from build123d import *

# Parameters (mm, degrees)
SKETCH1_R           = 251.5
BOSS_EXTRUDE1_DEPTH = 3
SKETCH2_R           = 2.5
CUT_EXTRUDE1_DEPTH  = 5
SKETCH4_R           = 2.5
CUT_EXTRUDE3_DEPTH  = 5
SKETCH5_W           = 73.96870399
SKETCH5_H           = 122
SKETCH5_W_2         = 122.237238898
SKETCH5_H_2         = 252
CUT_EXTRUDE4_DEPTH  = 10
FILLET1_R           = 2


with BuildPart() as part:
    # Sketch1 → Boss-Extrude1 (new body)
    with BuildSketch(Plane(origin=(0, 0, 0), x_dir=(1, 0, 0), z_dir=(0, 1, 0))):
        with Locations(Location((0, 0, 0), (0, 0, 270))):
            Circle(SKETCH1_R)
    extrude(amount=BOSS_EXTRUDE1_DEPTH)

    # Sketch2 → Cut-Extrude1 (cut)
    with BuildSketch(Plane(origin=(0, 3, 0), x_dir=(1, 0, 0), z_dir=(0, 1, 0))):
        with Locations(Location((-136, 118, 0), (0, 0, 270))):
            Circle(SKETCH2_R)
        with Locations(Location((136, 118, 0), (0, 0, 270))):
            Circle(SKETCH2_R)
        with Locations(Location((136, -118, 0), (0, 0, 270))):
            Circle(SKETCH2_R)
        with Locations(Location((-136, -118, 0), (0, 0, 270))):
            Circle(SKETCH2_R)
    extrude(amount=-CUT_EXTRUDE1_DEPTH, mode=Mode.SUBTRACT)

    # Sketch4 → Cut-Extrude3 (cut)
    with BuildSketch(Plane(origin=(0, 3, 0), x_dir=(1, 0, 0), z_dir=(0, 1, 0))):
        with Locations(Location((0, 242.5, 0), (0, 0, 270))):
            Circle(SKETCH4_R)
        with Locations(Location((142.537923681, 196.186621136, 0), (0, 0, 270))):
            Circle(SKETCH4_R)
        with Locations(Location((230.631205202, 74.936621136, 0), (0, 0, 270))):
            Circle(SKETCH4_R)
        with Locations(Location((230.631205202, -74.936621136, 0), (0, 0, 270))):
            Circle(SKETCH4_R)
        with Locations(Location((142.537923681, -196.186621136, 0), (0, 0, 270))):
            Circle(SKETCH4_R)
        with Locations(Location((0, -242.5, 0), (0, 0, 270))):
            Circle(SKETCH4_R)
        with Locations(Location((-142.537923681, -196.186621136, 0), (0, 0, 270))):
            Circle(SKETCH4_R)
        with Locations(Location((-230.631205202, -74.936621136, 0), (0, 0, 270))):
            Circle(SKETCH4_R)
        with Locations(Location((-230.631205202, 74.936621136, 0), (0, 0, 270))):
            Circle(SKETCH4_R)
        with Locations(Location((-142.537923681, 196.186621136, 0), (0, 0, 270))):
            Circle(SKETCH4_R)
    extrude(amount=-CUT_EXTRUDE3_DEPTH, mode=Mode.SUBTRACT)

    # Sketch5 → Cut-Extrude4 (cut)
    with BuildSketch(Plane(origin=(0, 3, 0), x_dir=(1, 0, 0), z_dir=(0, 1, 0))):
        with Locations((-225.484351995, 0)):
            Rectangle(SKETCH5_W, SKETCH5_H)
        with Locations((225.618619449, 0)):
            Rectangle(SKETCH5_W_2, SKETCH5_H_2)
    extrude(amount=-CUT_EXTRUDE4_DEPTH, mode=Mode.SUBTRACT)

    # Fillet1
    fillet1_edges = [part.edges().sort_by_distance(p)[0] for p in [
        (-188.5, 1.5, -61),
        (-243.990266199, 1.5, 61),
        (-188.5, 1.5, 61),
        (-243.990266199, 1.5, -61),
        (164.5, 1.5, 126),
        (217.660860055, 1.5, -126),
        (164.5, 1.5, -126),
        (217.660860055, 1.5, 126),
    ]]
    fillet(fillet1_edges, radius=FILLET1_R)


solid = part.part
Source: CAD feature listing. Evaluate the final solid. Frame: model axes, mm. Give positions to 0.01 mm unless a question says otherwise; leave off trailing zeros. Write each loop counter-clockwise with the first axis right and the second up, starting at its lowest first coordinate (ties: lowest second). Pieces come first, ordered by that corner, then holes. Notation, with made-up numbers: (8.5, 39) -> (66.5, 39) arc R33 ccw to (66.5, 75) -> close; hole circle Ø10 at (-17.5, 7.25). An arc over 180 degrees is marked (long way). Write item = value, one per line.
Q1. Cut plane A-A on y = 1.8. State how many separate pieces and enclosed holes the cut face has, then the cut area to 3 significant figures.
Here are the results:
separate_pieces = 1
enclosed_holes = 12
area = 172,000 mm²
Q2. Mould query, pull axis Y, two halves, no side actions, for faces 1 (the face through (-10, 0, -4)), 2 (the face through (-39.61, 1.48, 248.36)), 3 (the face through (-10, 3, -4)). Classes: +Y half, -Y half, draft (parallel to the pull), parting line (faces both ways), or undercut.
Here are the results:
face_1 = -Y half
face_2 = draft
face_3 = +Y half
Q3. Cut plane C-C on z = -27. Return loops of the section in (x, y), then the cut area to 3 significant figures.
Here are the results:
outline = (-188.5, 0) -> (164.5, 0) -> (164.5, 3) -> (-188.5, 3) -> close
area = 1,060 mm²
Q4. Cut plane B-B on x = 126.5. Return loops of the section in (y, z), then the cut area to 3 significant figures.
Here are the results:
outline = (0, -217.37) -> (3, -217.37) -> (3, 217.37) -> (0, 217.37) -> close
area = 1,300 mm²
Q5. First-contact query: pin 1 (0.9 mm diameter, centred on x = -220.5, y = 1.5, fed in from -Z); pin 2 (0.9 mm diameter, centred on x = 183, y = 2, fed in from +Z); pin 3 (1.5 mm diameter, centred on x = -219.5, y = 1.5, fed in from +Z). Flat tips, straight axial feed; report the tip coordinate or a pass-through.
Here are the results:
pin_1 = -121.78
pin_2 = 173
pin_3 = 124.1
Q6. Line query: line 1 (Z direction, x = 136, y = 2.25); line 2 (X direction, y = 1.8, z = -40); line 3 (X direction, y = 2.35, z = -118). Output: solid intervals per line, ascending. Write a range as from..to.
Here are the results:
line_1 = -211.56..-120.5, -115.5..115.5, 120.5..211.56
line_2 = -188.5..164.5
line_3 = -222.1..-138.5, -133.5..133.5, 138.5..164.5
